Build history of the part. All positions in model axes, mm. A direction names the side the tool comes from. Coordinates: 2 decimals unless noted, no trailing zeros. Order: outer loops, then holes, each group sorted by start corner. A loop starts at its lowest first (then second) coordinate and runs counter-clockwise, first axis right, second up. Notation, with made-up numbers: (70, 69.25) - (104, 69.25) arc R20 cw to (104, 106.25) - close; hole circle Ø11 at (23.5, 29). An arc over 180 degrees is marked (long way). Return JSON: item names as keys, results as strings.
from build123d import *

# Parameters (mm, degrees)
SKETCH1_W           = 110
SKETCH1_H           = 90
BOSS_EXTRUDE1_DEPTH = 5
SKETCH4_W           = 105.4
SKETCH4_H           = 85.4
SKETCH4_W_2         = 101.4
SKETCH4_H_2         = 81.4
BOSS_EXTRUDE2_DEPTH = 20
SKETCH5_R           = 5
BOSS_EXTRUDE3_DEPTH = 7
SKETCH6_R           = 3
CUT_EXTRUDE1_DEPTH  = 5


with BuildPart() as part:
    # Sketch1 → Boss-Extrude1 (new body)
    with BuildSketch(Plane(origin=(0, 0, 0), x_dir=(1, 0, 0), z_dir=(0, 1, 0))):
        Rectangle(SKETCH1_W, SKETCH1_H)
    extrude(amount=BOSS_EXTRUDE1_DEPTH)

    # Sketch4 → Boss-Extrude2 (add)
    with BuildSketch(Plane(origin=(0, 5, 0), x_dir=(1, 0, 0), z_dir=(0, 1, 0))):
        Rectangle(SKETCH4_W, SKETCH4_H)
        Rectangle(SKETCH4_W_2, SKETCH4_H_2, mode=Mode.SUBTRACT)
    extrude(amount=BOSS_EXTRUDE2_DEPTH)

    # Sketch5 → Boss-Extrude3 (add)
    with BuildSketch(Plane(origin=(0, 5, 0), x_dir=(1, 0, 0), z_dir=(0, 1, 0))):
        with Locations((-40.380300674, 32.341761364)):
            Circle(SKETCH5_R)
        with Locations((-40.380300674, -30.658238636)):
            Circle(SKETCH5_R)
        with Locations((42.619699326, -30.658238636)):
            Circle(SKETCH5_R)
        with Locations((42.619699326, 32.341761364)):
            Circle(SKETCH5_R)
    extrude(amount=BOSS_EXTRUDE3_DEPTH)

    # Sketch6 → Cut-Extrude1 (cut)
    with BuildSketch(Plane(origin=(0, 12, 0), x_dir=(1, 0, 0), z_dir=(0, 1, 0))):
        with Locations((-40.380300674, 32.341761364)):
            Circle(SKETCH6_R)
        with Locations((-40.380300674, -30.658238636)):
            Circle(SKETCH6_R)
        with Locations((42.619699326, -30.658238636)):
            Circle(SKETCH6_R)
        with Locations((42.619699326, 32.341761364)):
            Circle(SKETCH6_R)
    extrude(amount=-CUT_EXTRUDE1_DEPTH, mode=Mode.SUBTRACT)


solid = part.part
1. Cut at B-B on x = -14.5. Give the cut face in (y, z).
Check values:
{"outline": "(0, -45) - (5, -45) - (5, -42.7) - (25, -42.7) - (25, -40.7) - (5, -40.7) - (5, 40.7) - (25, 40.7) - (25, 42.7) - (5, 42.7) - (5, 45) - (0, 45) - close"}
2. Cut at A-A on y = 8.75. State how many separate pieces and enclosed holes the cut face has, plus the area to 3 significant figures.
Check values:
{"separate pieces": "5", "enclosed holes": "5", "area": "948 mm²"}
3. Tool access for faces 1 (the flat face through (-52.7, 15, 1)), 2 (the flat face through (52.7, 15, 1)), 3 (the flat face through (-1, 15, -42.7)), 4 (the cylindrical face through (41.969, 9.535, 33.587)): list every direction of +Z, -Z, +X, -X, +Y, -Y with a clear straight run to the whole face (end or side of a thin tool).
Check values:
{"face 1": "+Z, -Z, -X, +Y", "face 2": "+Z, -Z, +X, +Y", "face 3": "-Z, +X, -X, +Y", "face 4": "+Y"}
4. Probe L1, parallel to X at y = 13.5, z = 37.5; L2, parallel to Z at x = 50, y = 21.5; L3, parallel to Y at x = 5.5, z = 11. List the from-to ranges inside material, lowest first.
Check values:
{"L1": "-52.7 to -50.7, 50.7 to 52.7", "L2": "-42.7 to -40.7, 40.7 to 42.7", "L3": "0 to 5"}
5. Cut at D-D on z = -6. Give the cut face in (x, y).
Check values:
{"outline": "(-55, 0) - (55, 0) - (55, 5) - (52.7, 5) - (52.7, 25) - (50.7, 25) - (50.7, 5) - (-50.7, 5) - (-50.7, 25) - (-52.7, 25) - (-52.7, 5) - (-55, 5) - close"}
6. Drop flat-ended pins along their axis: pin 1 (9.5 mm diameter, centred on x = 42.62, z = -32.34, fed in from +Y); pin 2 (6 mm diameter, centred on y = 14.5, z = -32, fed in from +X); pin 3 (5.5 mm diameter, centred on x = -40.38, z = 30.66, fed in from +Y). Give the stop position or say it passes through.
Check values:
{"pin 1": "y = 12", "pin 2": "x = 52.7", "pin 3": "y = 7"}
7. Cut at C-C on y = 21.5. Give the cut face in (x, z), plus the area to 3 significant figures.
Check values:
{"outline": "(-52.7, -42.7) - (52.7, -42.7) - (52.7, 42.7) - (-52.7, 42.7) - close; hole (-50.7, -40.7) - (50.7, -40.7) - (50.7, 40.7) - (-50.7, 40.7) - close", "area": "747 mm²"}
